CAD build for the part. Positions are in the model's coordinates, mm. A direction names the side the tool comes from. Round coordinates to 2 decimals unless told otherwise and drop trailing zeros.
```python
from build123d import *

# Parameters (mm, degrees)
F0_R     = 73.025
F1_DEPTH = 25.4
F2_R     = 41.275
F3_DEPTH = 101.6
F4_R     = 20.32
F5_DEPTH = 127.001
F6_R     = 5.55625
F6_R_2   = 34.925
F7_DEPTH = 76.2
F8_SIZE  = 3.175


with BuildPart() as f1:
    # F0 (on Top) → F1 (new body)
    with BuildSketch(Plane.XY):
        Circle(F0_R)
    extrude(amount=F1_DEPTH)

    # F2 (on face) → F3 (join)
    with BuildSketch(Plane(origin=(0, 0, 0), x_dir=(1, 0, 0), z_dir=(0, 0, -1))):
        Circle(F2_R)
    extrude(amount=F3_DEPTH)

    # F4 (on face) → F5 (cut, through all)
    with BuildSketch(Plane(origin=(0, 0, -101.6), x_dir=(1, 0, 0), z_dir=(0, 0, -1))):
        Circle(F4_R)
    extrude(amount=-F5_DEPTH, mode=Mode.SUBTRACT)

    # F6 (on face) → F7 (cut)
    with BuildSketch(Plane.XY.offset(25.4)):
        with Locations((-57.15, 0)):
            Circle(F6_R)
        with Locations((0, 57.15)):
            Circle(F6_R)
        with Locations((57.15, 0)):
            Circle(F6_R)
        with Locations((0, -57.15)):
            Circle(F6_R)
        Circle(F6_R_2)
    extrude(amount=-F7_DEPTH, mode=Mode.SUBTRACT)

    # F8
    f8_edges = [f1.edges().sort_by_distance(p)[0] for p in [
        (-73.025, 0, 25.4),
        (-73.025, 0, 0),
        (-41.275, 0, -101.6),
    ]]
    chamfer(f8_edges, length=F8_SIZE)


solid = f1.part
```
Item 1: 3-axis set-ups, long thin cutter, end or side, ignore diameter. For faces 4 (the cylindrical face through (69.653, 21.935, 12.567)), 5 (the flat face through (30, -30, 0)), 6 (the flat face through (15, -15, -50.8)): which of +Z, -Z, +X, -X, +Y, -Y reach the whole face in a straight line?
Answers follow:
face 4: +Z, -Z
face 5: -Z
face 6: +Z
Item 2: Probe line 1 (Y direction, x = 0, z = 17) (3 decimals); line 2 (Z direction, x = -24, y = 62); line 3 (Y direction, x = 20.5, z = 10). List the from-to ranges inside material, lowest first.
Answers follow:
line 1: y = -73.025 to -62.706, -51.594 to -34.925, 34.925 to 51.594, 62.706 to 73.025
line 2: z = 0 to 25.4
line 3: y = -70.09 to -28.28, 28.28 to 70.09
Item 3: Flat gauge pins, fed straight in: P1, Ø12, axis at x = 6, y = -56.5, coming from the -Z side; P2, Ø21, axis at x = -17, y = 0, coming from the +Z side; P3, Ø2, axis at y = 7, z = -76.5, coming from the -X side; P4, Ø6, axis at x = -28, y = 18.5, coming from the +Z side. Where does each tip first touch, or does it go through?
Answers follow:
P1: stops at z = 0
P2: stops at z = -50.8
P3: stops at x = -40.84
P4: stops at z = 25.4
Item 4: Cut at A-A, the plane x = 0. State how many separate pieces and enclosed holes the cut face has, plus the area to 3 significant figures.
Answers follow:
separate pieces: 4
enclosed holes: 0
area: 4,110 mm2
Item 5: Two-plate mould, pull along X, no slides. Class faces 1 (the flat face through (16, 16, -101.6)), 2 (the conical face through (36.488, -11.491, -101.446)), 3 (the cylindrical face through (-27.715, -21.251, -12.167)): released by +X, released by -X, zero draft, split by the parting line, or undercut.
Answers follow:
face 1: zero draft
face 2: split by the parting line
face 3: undercut
